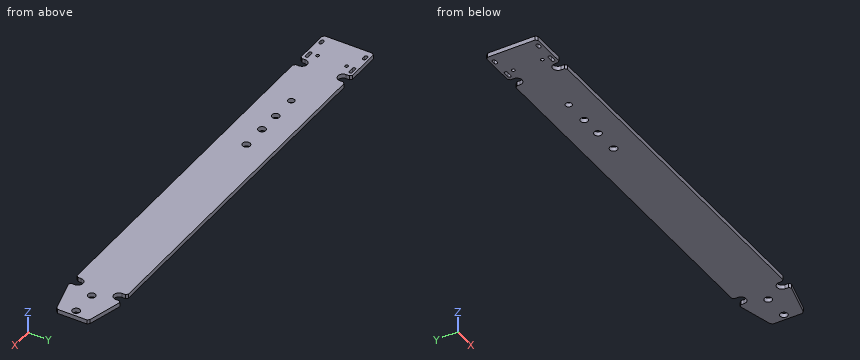
from build123d import *

# Parameters (mm, degrees)
EXTRUDE_1_OUTLINE_R = 0.325
EXTRUDE_1_DEPTH     = 0.85
SKETCH_1_R          = 0.635
SKETCH_1_R_2        = 0.750616105
CUT_EXTRUDE_1_DEPTH = 92.204552414


# Read off the part's stored shape, not the designer's step: 凸台-拉伸1
with BuildPart() as part:
    # 凸台-拉伸1 outline → 凸台-拉伸1 (new body)
    with BuildSketch(Plane.XY):
        with BuildLine():
            Line((81.153, -5.08), (81.534, -4.699))
            Line((81.534, -4.699), (81.534, -4.064))
            ThreePointArc((81.534, -4.064), (82.55, -3.048), (83.566, -4.064))
            Line((83.566, -4.064), (83.566, -4.699))
            Line((83.566, -4.699), (83.947, -5.08))
            Line((83.947, -5.08), (90.678, -3.3))
            Line((90.678, -3.3), (91.059, -2.919))
            Line((91.059, -2.919), (91.059, 0))
            Line((91.059, 0), (1.27, 0))
            Line((1.27, 0), (1.27, -4.699))
            Line((1.27, -4.699), (1.651, -5.08))
            Line((1.651, -5.08), (8.382, -5.08))
            Line((8.382, -5.08), (8.763, -4.699))
            Line((8.763, -4.699), (8.763, -4.064))
            ThreePointArc((8.763, -4.064), (9.779, -3.048), (10.795, -4.064))
            Line((10.795, -4.064), (10.795, -4.699))
            Line((10.795, -4.699), (11.176, -5.08))
            Line((11.176, -5.08), (81.153, -5.08))
        make_face()
        with BuildLine():
            Line((2.728, -4.02), (3.348, -4.02))
            ThreePointArc((3.348, -4.02), (3.648, -4.32), (3.348, -4.62))
            Line((3.348, -4.62), (2.728, -4.62))
            ThreePointArc((2.728, -4.62), (2.428, -4.32), (2.728, -4.02))
        make_face(mode=Mode.SUBTRACT)
        with BuildLine():
            Line((7.763, -4.62), (6.663, -4.62))
            ThreePointArc((6.663, -4.62), (6.363, -4.32), (6.663, -4.02))
            Line((6.663, -4.02), (7.763, -4.02))
            ThreePointArc((7.763, -4.02), (8.063, -4.32), (7.763, -4.62))
        make_face(mode=Mode.SUBTRACT)
        with Locations((6.683, -2.8687)):
            Circle(EXTRUDE_1_OUTLINE_R, mode=Mode.SUBTRACT)
    extrude_1 = extrude(amount=EXTRUDE_1_DEPTH)

    # 镜向1: 凸台-拉伸1 across plane
    add(extrude_1.mirror(Plane(origin=(0, 0, 0.85), x_dir=(0, 0, 1), z_dir=(0, 1, 0))))

    # 草图1 → 切除-拉伸1 (cut, through all)
    with BuildSketch(Plane.XY):
        with Locations((19.914, 0)):
            Circle(SKETCH_1_R)
        with Locations((24.994, 0)):
            Circle(SKETCH_1_R_2)
        with Locations((29.414, 0)):
            Circle(SKETCH_1_R_2)
        with Locations((34.494, 0)):
            Circle(SKETCH_1_R_2)
        with Locations((89.789, 0)):
            Circle(SKETCH_1_R_2)
        with Locations((84.709, 0)):
            Circle(SKETCH_1_R_2)
    extrude(amount=CUT_EXTRUDE_1_DEPTH, mode=Mode.SUBTRACT)


solid = part.part
Can you work these out from the model? Positions are in its coordinate system, mm. Round coordinates to 2 decimals unless told otherwise and drop trailing zeros. Order: outer loops, then holes, each group sorted by start corner. A loop starts at its lowest first (then second) coordinate and runs counter-clockwise, first axis right, second up. Notation, with made-up numbers: M 61,35 L 76,35 A27 ccw 76,61 Z; hole C 54,-35 d4. An arc over 180 degrees is marked long. Use a Markdown table: item, result.
1) Imagine slicing it at B-B (z = 0.55). Give the number of separate pieces and of enclosed holes in the cut face, then the cut area to 3 significant figures.
Geometry says:
| item | result |
|---|---|
| separate pieces | 1 |
| enclosed holes | 12 |
| area | 869 mm² |
2) Imagine slicing it at C-C (x = 82.55). List the corners of the cut face in (y, z) for me.
Geometry says:
| item | result |
|---|---|
| outline | M -3.05,0 L 3.05,0 L 3.05,0.85 L -3.05,0.85 Z |
3) If I drill on line 1 along X through (y, z) = (-2.75, 0.5); line 2 along X through (y, z) = (3.25, 0.15); line 3 along Y through (x, z) = (86.5, 0.4), over which ranges is the centre line in solid material (lowest first)?
Geometry says:
| item | result |
|---|---|
| line 1 | x = 1.27 to 6.38, 6.99 to 91.06 |
| line 2 | x = 1.27 to 9.17, 10.39 to 81.94, 83.16 to 90.73 |
| line 3 | y = -4.4 to 4.4 |
4) Imagine slicing it at A-A (x = 25). List the corners of the cut face in (y, z) for me, then the cut area to 3 significant figures.
Geometry says:
| item | result |
|---|---|
| outline | M -5.08,0 L -0.75,0 L -0.75,0.85 L -5.08,0.85 Z; M 0.75,0 L 5.08,0 L 5.08,0.85 L 0.75,0.85 Z |
| area | 7.36 mm² |
